Here's how the part is built. I have some questions about the finished solid (model axes, mm). Face numbers are marked on the shaded views. Give positions to 0.01 mm unless a question says otherwise; leave off trailing zeros. Write each loop counter-clockwise with the first axis right and the second up, starting at its lowest first coordinate (ties: lowest second). Pieces come first, ordered by that corner, then holes. Notation, with made-up numbers: (-23, -37) -> (1, -37) arc R26 cw to (1, 2) -> close; hole circle Ø6 at (75, 75.25). An arc over 180 degrees is marked (long way). Use CSV: the item, a comma, the result in double quotes. Start each with the question number.
(1) For pin 1 Ø3.5 at (x, z) = (0, 40) entering from +Y; pin 2 Ø1.5 at (x, z) = (-18, -17.5) entering from +Y; pin 3 Ø4 at (x, z) = (-40, 0) entering from -Y; pin 4 Ø1 at (x, y) = (-31, 2) entering from +Z, each with a flat end and sliding along its axis, tell me the tip position at first contact or that it passes through.
(2) Suppose I cut it at D-D on z = 25. List the corners of the cut face in (x, y) for me.
(3) I need wall thicknesses on L1, parallel to X at y = 8, z = 0; L2, parallel to Z at x = 0, y = 0.3; L3, parallel to X at y = 1.4, z = 0. Which ranges of each line are inside material? Lowest first, please. Write a range as [from, to].
(4) Suppose I cut it at A-A on z = 0. Give the number of separate pieces and of enclosed holes in the cut face, plus the area to 3 significant figures.
(5) If we mould it in two halves opening along Z, with no side actions, what happens to the marked faces 1, 2 and 3? For each: pulls with the +Z half, pulls with the -Z half, needs draft (parallel to the pull), parting line crosses it, or undercut.
(6) Suppose I cut it at B-B on x = -7. List the corners of the cut face in (y, z) for me.
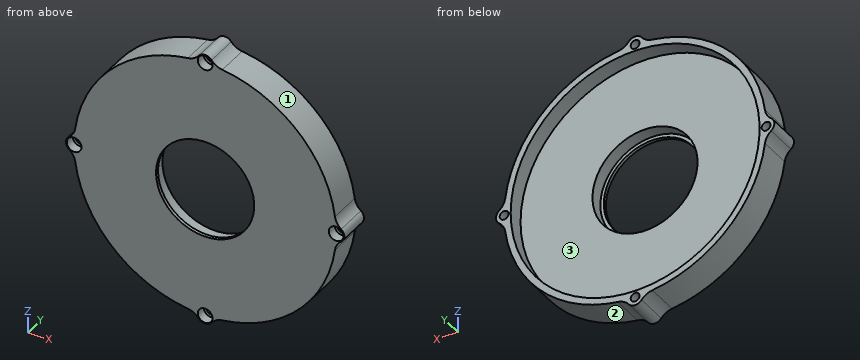
Autodesk Inventor part; units mm, degrees
ref_plane "YZ Plane" through (0, 0, 0) normal (1, 0, 0) x (0, 1, 0)
ref_plane "XZ Plane" through (0, 0, 0) normal (0, 1, 0) x (-1, 0, 0)
ref_plane "XY Plane" through (0, 0, 0) normal (0, 0, 1) x (1, 0, 0)
sketch "Szkic1" plane through (0, 0, 0) normal (0, 1, 0) x (-1, 0, 0)
  circle A0 centre (0, 0) radius 40
  circle A1 centre (0, 0) radius 15
  dimension "d0" = 80
  dimension "d1" = 30
extrude "Wyciągnięcie proste1" add sketch "Szkic1" along normal blind 1
sketch "Szkic2" plane through (0, 1, 0) normal (0, 1, 0) x (1, 0, 0)
  circle A0 centre (0, 0) radius 40
  circle A1 centre (0, 0) radius 16.05
  dimension "d4" = 32.1
extrude "Wyciągnięcie proste2" add sketch "Szkic2" along normal blind 4
sketch "Szkic3" plane through (0, 5, 0) normal (0, 1, 0) x (1, 0, 0)
  circle A0 centre (0, 0) radius 40
  circle A1 centre (0, 0) radius 38
  dimension "d7" = 76
extrude "Wyciągnięcie proste3" add sketch "Szkic3" along normal blind 5
sketch "Szkic4" plane through (0, 0, 0) normal (0, -1, 0) x (1, 0, 0)
  circle A0 centre (0, 0) radius 40
  circle A1 centre (0, 40) radius 1.35
  circle A2 centre (0, 40) radius 2.5
  point P0 (2.4988, 39.9219)
  point P1 (-2.4988, 39.9219)
  dimension "d10" = 2.7
  dimension "d11" = 5
extrude "Wyciągnięcie proste4" add sketch "Szkic4" against normal blind 10 contours A0 A1 A2 | A0 A1 picked at (1.9426, 40.8023) picked at (0.0508, 40.4454)
fillet "Zaokrąglenie1" radius 5 4 edges at (2.4988, 0.5, 39.9219) (2.4988, 5.5, 39.9219) (-2.4988, 5.5, 39.9219) (-2.4988, 0.5, 39.9219)
sketch "Szkic5" plane through (0, 0, 0) normal (0, -1, 0) x (1, 0, 0)
  circle A0 centre (0, 40) radius 1.35
  point P0 (0, 0)
  dimension "d15" = 2.7
extrude "Wyciągnięcie proste5" cut sketch "Szkic5" against normal blind 10
sketch "Szkic6" plane through (0, 0, 0) normal (0, -1, 0) x (1, 0, 0)
  circle A0 centre (0, 40) radius 1.35
  circle A1 centre (0, 40) radius 2.25
  point P0 (0, 0)
  dimension "d18" = 4.5
extrude "Wyciągnięcie proste6" cut sketch "Szkic6" against normal blind 3
pattern_circular "Szyk kołowy1" count 4 over 360 about axis through (0, 0, 0) along (0, 1, 0) of "Wyciągnięcie proste5", "Wyciągnięcie proste6", "Zaokrąglenie1", "Wyciągnięcie proste4"
properties part number "End"
Geometry says:
1,pin 1,"y = 10"
1,pin 2,"y = 5"
1,pin 3,"y = 3"
1,pin 4,"z = 25.88"
2,outline,"(-31.22, 0) -> (31.22, 0) -> (31.22, 10) -> (28.62, 10) -> (28.62, 5) -> (-28.62, 5) -> (-28.62, 10) -> (-31.22, 10) -> close"
3,L1,"[-42.5, -41.35], [-38.65, -38], [38, 38.65], [41.35, 42.5]"
3,L2,"[-42.5, -42.25], [-37.75, -15], [15, 37.75], [42.25, 42.5]"
3,L3,"[-42.5, -42.25], [-37.75, -16.05], [16.05, 37.75], [42.25, 42.5]"
4,separate pieces,"4"
4,enclosed holes,"0"
4,area,"247 mm²"
5,face 1,"pulls with the +Z half"
5,face 2,"pulls with the -Z half"
5,face 3,"undercut"
6,outline,"(0, -39.38) -> (10, -39.38) -> (10, -37.35) -> (5, -37.35) -> (5, -14.44) -> (1, -14.44) -> (1, -13.27) -> (0, -13.27) -> close; (0, 13.27) -> (1, 13.27) -> (1, 14.44) -> (5, 14.44) -> (5, 37.35) -> (10, 37.35) -> (10, 39.38) -> (0, 39.38) -> close"
